from build123d import *

# Parameters (mm, degrees)
SKETCH1_W      = 152.4
SKETCH1_H      = 152.4
SKETCH1_R      = 9.525
EXTRUDE1_DEPTH = 9.525
SKETCH3_R      = 44.45
FILLET1_R      = 9.525


with BuildPart() as part:
    # Sketch1 → Extrude1 (new body)
    with BuildSketch(Plane(origin=(0, 0, 0), x_dir=(0, 0, -1), z_dir=(1, 0, 0))):
        Rectangle(SKETCH1_W, SKETCH1_H)
        with Locations(Location((-53.975, 53.975, 0), (0, 0, 180))):
            Circle(SKETCH1_R, mode=Mode.SUBTRACT)
        with Locations(Location((-53.975, -53.975, 0), (0, 0, 180))):
            Circle(SKETCH1_R, mode=Mode.SUBTRACT)
        with Locations(Location((53.975, -53.975, 0), (0, 0, 180))):
            Circle(SKETCH1_R, mode=Mode.SUBTRACT)
        with Locations(Location((53.975, 53.975, 0), (0, 0, 180))):
            Circle(SKETCH1_R, mode=Mode.SUBTRACT)
    extrude(amount=EXTRUDE1_DEPTH)

    # Sweep1: sweep along a path in Sketch2
    with BuildLine(Plane.XY) as sweep1_path:
        ThreePointArc((9.525, 0), (167.301089894, -20.771616294), (314.325, -81.670913853))
    # Sketch3 → Sweep1 (sweep)
    with BuildSketch(Plane(origin=(9.525, 0, 0), x_dir=(0, 0, -1), z_dir=(1, 0, 0))):
        Circle(SKETCH3_R)
    sweep(path=sweep1_path.line)

    # Fillet1
    fillet1_edges = [part.edges().sort_by_distance(p)[0] for p in [
        (9.525, 0, 44.45),
    ]]
    fillet(fillet1_edges, radius=FILLET1_R)


solid = part.part
Check sheet for the modelled part. Datum: model origin and axes. Units: mm. A direction names the side the tool comes from. Round coordinates to 2 decimals unless told otherwise and drop trailing zeros.
Q1. Draft check along Y on faces 3 (the face through (4.7, -60.41, -61)), 4 (the face through (4.7, -60.41, 46.95)), 5 (the face through (9.525, 52, 18)), 6 (the face through (5, 76.2, 1)). Enter one of: pulls with the +Y half, pulls with the -Y half, needs draft (parallel to the pull), parting line crosses it, or undercut.
Filled sheet:
face 3: undercut
face 4: undercut
face 5: needs draft
face 6: pulls with the +Y half
Q2. Depth check by flat-ended pin: P1, Ø8, axis at x = 72, z = 36, coming from the +Y side; P2, Ø5, axis at y = -87, z = -21, coming from the +X side; P3, Ø8, axis at y = -55, z = -55.5, coming from the +X side; P4, Ø3, axis at y = -76, z = 56, coming from the +X side (3 decimals). Enter the tip coordinate at first touch or a pass-through.
Filled sheet:
P1: stops at y = 27.82
P2: stops at x = 312.69
P3: passes through
P4: stops at x = 9.525
Q3. Set-up check for faces 1 (the face through (4.696, 59.771, -61.534)), 2 (the face through (5, -76.2, 1)): record each of +Z, -Z, +X, -X, +Y, -Y from which the full face is reachable in a straight line by a thin tool's end or side.
Filled sheet:
face 1: +X, -X
face 2: +Z, -Z, -X, -Y
Q4. Scan lines: L1, parallel to X at y = 45, z = 67 (3 decimals); L2, parallel to Z at x = 172, y = -24; L3, parallel to Z at x = 201, y = -36. Record each from-to range of solid material in increasing order.
Filled sheet:
L1: x = 0 to 9.525
L2: z = -44.41 to 44.41
L3: z = -44.18 to 44.18
